from build123d import *

# Parameters (mm, degrees)
EXTRUDE_1_DEPTH     = 2
SKETCH_11_W         = 4.2
SKETCH_11_H         = 15
SKETCH_11_W_2       = 16.8
SKETCH_11_H_2       = 22
SKETCH_11_W_3       = 5
SKETCH_11_R         = 3.5
SKETCH_11_R_2       = 1.5
CUT_EXTRUDE_1_DEPTH = 10
FILLET_1_R          = 5


with BuildPart() as part:
    # Эскиз1 → Бобышка-Вытянуть1 (new, symmetric)
    with BuildSketch(Plane.XY):
        with BuildLine():
            Line((-90, 15), (90, 15))
            ThreePointArc((90, 15), (105, 0), (90, -15))
            Line((90, -15), (-90, -15))
            ThreePointArc((-90, -15), (-105, 0), (-90, 15))
        make_face()
    extrude(amount=EXTRUDE_1_DEPTH, both=True)

    # Эскиз11 → Вырез-Вытянуть1 (cut)
    with BuildSketch(Plane(origin=(0, 0, -2), x_dir=(-1, 0, 0), z_dir=(0, 0, -1))):
        with Locations((-87.9, 7.5)):
            Rectangle(SKETCH_11_W, SKETCH_11_H)
        with Locations((-73.4, 0)):
            Rectangle(SKETCH_11_W_2, SKETCH_11_H_2)
        with Locations((-57.5, 0)):
            Rectangle(SKETCH_11_W_3, SKETCH_11_H_2)
        with Locations((-47.5, 0)):
            Rectangle(SKETCH_11_W_3, SKETCH_11_H_2)
        with Locations((-37.5, 0)):
            Rectangle(SKETCH_11_W_3, SKETCH_11_H_2)
        with Locations((-27.5, 0)):
            Rectangle(SKETCH_11_W_3, SKETCH_11_H_2)
        with Locations((-17.5, 0)):
            Rectangle(SKETCH_11_W_3, SKETCH_11_H_2)
        with Locations((-7.5, 0)):
            Rectangle(SKETCH_11_W_3, SKETCH_11_H_2)
        with Locations((7.5, 0)):
            Rectangle(SKETCH_11_W_3, SKETCH_11_H_2)
        with Locations((17.5, 0)):
            Rectangle(SKETCH_11_W_3, SKETCH_11_H_2)
        with Locations((27.5, 0)):
            Rectangle(SKETCH_11_W_3, SKETCH_11_H_2)
        with Locations((37.5, 0)):
            Rectangle(SKETCH_11_W_3, SKETCH_11_H_2)
        with Locations((47.5, 0)):
            Rectangle(SKETCH_11_W_3, SKETCH_11_H_2)
        with Locations((57.5, 0)):
            Rectangle(SKETCH_11_W_3, SKETCH_11_H_2)
        with Locations((73.4, 0)):
            Rectangle(SKETCH_11_W_2, SKETCH_11_H_2)
        with Locations((87.9, 7.5)):
            Rectangle(SKETCH_11_W, SKETCH_11_H)
        with Locations((97, 0)):
            Circle(SKETCH_11_R)
        with Locations((-97, 0)):
            Circle(SKETCH_11_R)
        Circle(SKETCH_11_R_2)
        with Locations((-90, -8)):
            Circle(SKETCH_11_R_2)
        with Locations((90, -8)):
            Circle(SKETCH_11_R_2)
    extrude(amount=-CUT_EXTRUDE_1_DEPTH, mode=Mode.SUBTRACT)

    # Скругление1
    fillet_1_edges = [part.edges().sort_by_distance(p)[0] for p in [
        (-65, 11, 0),
        (-81.8, 11, 0),
        (-81.8, -11, 0),
        (-65, -11, 0),
        (65, 11, 0),
        (65, -11, 0),
        (81.8, -11, 0),
        (81.8, 11, 0),
    ]]
    fillet(fillet_1_edges, radius=FILLET_1_R)


solid = part.part
The model under review builds one solid part; all positions refer to its coordinate system, in mm. A direction names the side the tool comes from. Coordinates: 2 decimals unless noted, no trailing zeros. Write each loop counter-clockwise with the first axis right and the second up, starting at its lowest first coordinate (ties: lowest second). Pieces come first, ordered by that corner, then holes. Notation, with made-up numbers: M 84,-30 L 143,-30 A27 cw 143,5 Z; hole C -9.5,-6 d9. An arc over 180 degrees is marked long. Put each result on its own line as item: value.
1) Wall thickness on probe 1 along Y at (x, z) = (25.5, 1.7); probe 2 along Y at (x, z) = (0, -1.75); probe 3 along Y at (x, z) = (-87, 1.4): over which ranges is each line inside the solid? List them lowest first. Write a range as [from, to].
Computed:
probe 1: y = [-15, -11], [11, 15]
probe 2: y = [-15, -1.5], [1.5, 15]
probe 3: y = [-15, 0]
2) Add section B-B on z = 0.7. State how many separate pieces and enclosed holes the cut face has, then the cut area to 3 significant figures.
Computed:
separate pieces: 1
enclosed holes: 19
area: 3,870 mm2
3) For faces 4 (the flat face through (1, 4, -2)), 5 (the flat face through (5, 0, 0)), list the 3-axis set-ups (+Z, -Z, +X, -X, +Y, -Y) from which the entire face can be reached by the end or side of a thin tool; tool diameter is ignored.
Computed:
face 4: -Z, +X, -X, +Y, -Y
face 5: +Z, -Z
4) Clearance check with flat-ended pins moving along their axes: pin 1 Ø2 at (y, z) = (-4, 0.5) entering from +X; pin 2 Ø1.2 at (y, z) = (-1, 0.5) entering from +X; pin 3 Ø1.2 at (y, z) = (10, 0) entering from -X; pin 4 Ø2.5 at (x, y) = (0, 0) entering from +Z. State where each tip first meets the part, or that it passes through.
Computed:
pin 1: stops at x = 104.7
pin 2: stops at x = 104.99
pin 3: stops at x = -101.69
pin 4: passes through
5) Add section A-A on x = 97. Give the boundary of the cut face in (y, z), then the cut area to 3 significant figures.
Computed:
outline: M -13.27,-2 L -3.5,-2 L -3.5,2 L -13.27,2 Z; M 3.5,-2 L 13.27,-2 L 13.27,2 L 3.5,2 Z
area: 78.1 mm2
6) Draft analysis for pull direction Y (two halves, no side actions). For faces 1 (the flat face through (-88, 0, 0)), 2 (the flat face through (8, -11, 0)), 3 (the flat face through (1, 4, 2)), state which applies: released by +Y, released by -Y, zero draft, split by the parting line, or undercut.
Computed:
face 1: released by +Y
face 2: undercut
face 3: zero draft
